For this review, take the finished solid that the model builds, in its own axes (mm). A direction names the side the tool comes from. Coordinates: 2 decimals unless noted, no trailing zeros. Write each loop counter-clockwise with the first axis right and the second up, starting at its lowest first coordinate (ties: lowest second). Pieces come first, ordered by that corner, then holes.
1) For faces 1 (the face through (-26, 150, -3.183)), 2 (the face through (0, 125, -13)), 3 (the face through (25, 265, -22.225)), list the 3-axis set-ups (+Z, -Z, +X, -X, +Y, -Y) from which the entire face can be reached by the end or side of a thin tool; tool diameter is ignored.
2) Insertion check: P1, Ø4, axis at x = -38.1, y = 228.6, coming from the +Z side (3 decimals); P2, Ø12.5, axis at x = 17, z = -13, coming from the -Y side; P3, Ø10, axis at y = 170.5, z = -4.5, coming from the +X side. Each pin has a flat end and moves straight along its axis. Give the tip position at first contact, or say it passes through.
3) We need section D-D on x = 7.5. Write out the cut boundary in (y, z) (3 decimals).
4) We need section B-B on x = 25.4. Write out the cut boundary in (y, z) (3 decimals).
5) We need section C-C on y = 25.4. Write out the cut boundary in (x, z) (3 decimals).
6) Mouldability with a two-part tool opening along Y and no side actions: class faces 4 (the face through (25, 257.175, -13)), 5 (the face through (0, 279, -13)), 6 (the face through (-25, 150, -22.225)), 7 (the face through (25, 254, -13)) as pulls with the +Y half, pulls with the -Y half, needs draft (parallel to the pull), parting line crosses it, or undercut.
7) We need section A-A on z = -13.25. Write out the cut boundary in (x, y) (3 decimals).
8) To check wall thickness, follow line 1 along Y through (x, z) = (-25.4, -23.05); line 2 along Z through (x, y) = (-25, 143.5) (3 decimals); line 3 along X through (y, z) = (46, -14.25) (3 decimals). State the ranges of each line that lie inside material, in increasing order.
Autodesk Inventor part; units mm, degrees
ref_plane "YZ Plane" through (0, 0, 0) normal (1, 0, 0) x (0, 1, 0)
ref_plane "XZ Plane" through (0, 0, 0) normal (0, 1, 0) x (-1, 0, 0)
ref_plane "XY Plane" through (0, 0, 0) normal (0, 0, 1) x (1, 0, 0)
sketch "Sketch1" plane through (0, 0, 0) normal (0, 1, 0) x (-1, 0, 0)
  line L0 (0, 0) -> (50.8, 0)
  line L1 (50.8, 0) -> (50.8, -25.4)
  line L2 (50.8, -25.4) -> (0, -25.4)
  line L3 (0, -25.4) -> (0, 0)
  line L4 (47.625, -3.1826) -> (3.175, -3.1826)
  line L5 (3.175, -3.1826) -> (3.175, -22.225)
  line L6 (3.175, -22.225) -> (47.625, -22.225)
  line L7 (47.625, -22.225) -> (47.625, -3.1826)
  dimension "d0" = 50.8
  dimension "d1" = 25.4
  dimension "d2" = 3.175
  dimension "d3" = 3.1826
  dimension "d4" = 3.175
  dimension "d5" = 3.175
extrude "Extrusion1" add sketch "Sketch1" along normal blind 304.8
sketch "Sketch2" plane through (0, 0, 0) normal (1, 0, 0) x (0, 0, -1)
  line L0 (25.4, 0) -> (25.4, 304.8)
  line L1 (0, 304.8) -> (25.4, 304.8)
  line L2 (25.4, 304.8) -> (25.4, 254)
  line L3 (25.4, 254) -> (0, 254)
  line L4 (0, 254) -> (0, 304.8)
  line L5 (3.1826, 0) -> (3.1826, 304.8)
  line L6 (3.1826, 301.7936) -> (22.225, 301.7936)
  line L7 (22.225, 301.7936) -> (22.225, 257.175)
  line L8 (22.225, 257.175) -> (3.1826, 257.175)
  line L9 (3.1826, 257.175) -> (3.1826, 301.7936)
  point P0 (0, 0)
  dimension "d8" = 50.8
  dimension "d9" = 3.175
  dimension "d10" = 3.175
extrude "Extrusion2" add sketch "Sketch2" along normal blind 50.8 contours L3 L5 L8 L7 L6 L1 L0 | L3 L4 L1 L5
sketch "Sketch3" plane through (0, 0, -25.4) normal (0, 0, -1) x (-1, 0, 0)
  circle A0 centre (-25.4, 280.6907) radius 14.2875
  line L0 (-50.8, 254) -> (-50.8, 304.8)
  point P0 (0, 0)
  dimension "d13" = 25.4
  dimension "d14" = 28.575
extrude "Extrusion3" cut sketch "Sketch3" against normal through all
sketch "Sketch4" plane through (0, 0, -25.4) normal (0, 0, -1) x (-1, 0, 0)
  circle A0 centre (24.6023, 25.4) radius 14.2875
  line L0 (50.8, 0) -> (0, 0)
  dimension "d17" = 25.4
  dimension "d18" = 28.575
extrude "Extrusion4" cut sketch "Sketch4" against normal up to next
sketch "Sketch5" plane through (0, 0, -25.4) normal (0, 0, -1) x (-1, 0, 0)
  circle A0 centre (25.4, 279.4) radius 14.2875
  line L0 (50.8, 304.8) -> (-50.8, 304.8)
  line L1 (50.8, 0) -> (50.8, 304.8)
  circle A1 centre (38.1, 228.6) radius 3.3734
  point P0 (0, 0)
  dimension "d21" = 25.4
  dimension "d22" = 28.575
  dimension "d23" = 25.4
  dimension "d32" = 6.7469
  dimension "d33" = 76.2
  dimension "d34" = 12.7
extrude "Extrusion5" cut sketch "Sketch5" against normal blind 25.4
sketch "Sketch6" plane through (-50.8, 0, 0) normal (0, 0, 1) x (1, 0, 0)
  line L0 (25.4, 18.0677) -> (19.05, 21.7338)
  line L1 (19.05, 21.7338) -> (19.05, 29.0662)
  line L2 (19.05, 29.0662) -> (25.4, 32.7323)
  line L3 (25.4, 32.7323) -> (31.75, 29.0662)
  line L4 (31.75, 29.0662) -> (31.75, 21.7338)
  line L5 (31.75, 21.7338) -> (25.4, 18.0677)
  line L6 (50.8, 0) -> (50.8, 254)
  line L7 (50.8, 0) -> (0, 0)
  point P0 (25.4, 25.4)
  dimension "d26" = 25.4
  dimension "d27" = 25.4
  dimension "d28" = 19.05
  dimension "d29" = 12.7
extrude "Extrusion6" cut sketch "Sketch6" against normal through all
properties part number "arm_new1" material "Aluminum 6061"
Result:
1. face 1: +Y, -Y
1. face 2: +Z, -Z, +X, -Y
1. face 3: +X
2. P1: passes through
2. P2: stops at y = 254
2. P3: stops at x = 0
3. outline: (254, -25.4) - (304.8, -25.4) - (304.8, 0) - (254, 0) - close; hole (257.175, -22.225) - (301.794, -22.225) - (301.794, -3.183) - (257.175, -3.183) - close
4. outline: (254, -25.4) - (266.403, -25.4) - (266.403, -22.225) - (257.175, -22.225) - (257.175, -3.183) - (266.403, -3.183) - (266.403, 0) - (254, 0) - close; (294.978, -25.4) - (304.8, -25.4) - (304.8, 0) - (294.978, 0) - (294.978, -3.183) - (301.794, -3.183) - (301.794, -22.225) - (294.978, -22.225) - close
5. outline: (-50.8, -25.4) - (-38.89, -25.4) - (-38.89, -22.225) - (-47.625, -22.225) - (-47.625, -3.183) - (-31.75, -3.183) - (-31.75, 0) - (-50.8, 0) - close; (-19.05, -3.183) - (-3.175, -3.183) - (-3.175, -22.225) - (-10.315, -22.225) - (-10.315, -25.4) - (0, -25.4) - (0, 0) - (-19.05, 0) - close
6. face 4: undercut
6. face 5: undercut
6. face 6: needs draft
6. face 7: pulls with the -Y half
7. outline: (-50.8, 0) - (-47.625, 0) - (-47.625, 304.8) - (-50.8, 304.8) - close; (-3.175, 0) - (0, 0) - (0, 254) - (50.8, 254) - (50.8, 257.175) - (0, 257.175) - (0, 301.794) - (50.8, 301.794) - (50.8, 304.8) - (-3.175, 304.8) - close
8. line 1: y = 0 to 11.13, 39.67 to 265.11, 293.69 to 304.8
8. line 2: z = -25.4 to -22.225, -3.183 to 0
8. line 3: x = -50.8 to -47.625, -3.175 to 0
